from build123d import *

# Parameters (mm, degrees)
SKIZZE1_W                       = 20
SKIZZE1_H                       = 40
AUFSATZ_LINEAR_AUSTRAGEN1_DEPTH = 300
SCHNITT_LINEAR_AUSTRAGEN1_DEPTH = 304.315017762


with BuildPart() as part:
    # Skizze1 → Aufsatz-Linear austragen1 (new body)
    with BuildSketch(Plane(origin=(0, 0, 0), x_dir=(1, 0, 0), z_dir=(0, 1, 0))):
        with Locations((10, 20)):
            Rectangle(SKIZZE1_W, SKIZZE1_H)
    extrude(amount=AUFSATZ_LINEAR_AUSTRAGEN1_DEPTH)

    # Skizze2 → Schnitt-Linear austragen1 (cut, through all)
    with BuildSketch(Plane(origin=(0, 300, 0), x_dir=(1, 0, 0), z_dir=(0, 1, 0))):
        Polygon((3, 30), (0, 33), (0, 27), align=None)
        Polygon((13, 40), (7, 40), (10, 37), align=None)
        Polygon((20, 27), (20, 33), (17, 30), align=None)
        Polygon((13, 20), (10, 17), (7, 20), align=None)
        Polygon((7, 20), (10, 23), (13, 20), align=None)
        Polygon((20, 7), (20, 13), (17, 10), align=None)
        Polygon((3, 10), (0, 13), (0, 7), align=None)
        Polygon((10, 3), (7, 0), (13, 0), align=None)
    extrude(amount=-SCHNITT_LINEAR_AUSTRAGEN1_DEPTH, mode=Mode.SUBTRACT)


solid = part.part
Could you check a few things on this model? Use its own coordinates, in mm. Coordinates: 2 decimals unless noted, no trailing zeros. Loops run counter-clockwise (first coordinate to the right, second up) from the corner with the lowest first, then second, coordinate; pieces in that order, holes last.
1. I need wall thicknesses on L1, parallel to X at y = 138, z = -20; L2, parallel to Z at x = 1.75, y = 84.5; L3, parallel to Z at x = 8, y = 120.5. Which ranges of each line are inside material? Lowest first, please.
2. For P1, Ø1, axis at x = 9.5, y = 89, coming from the +Z side; P2, Ø1, axis at x = 8.5, y = 57, coming from the +Z side, each with a flat end and sliding along its axis, tell me the tip position at first contact or that it passes through.
3. Imagine slicing it at A-A (y = 276.5). Please give me the cut outline in (x, z), and give its area (3 significant figures).
Computed values:
1. L1: x = 0 to 7, 13 to 20
1. L2: z = -40 to -31.25, -28.75 to -11.25, -8.75 to 0
1. L3: z = -39 to -21, -19 to -1
2. P1: stops at z = -2
2. P2: stops at z = -1
3. outline: (0, -40) - (7, -40) - (10, -37) - (13, -40) - (20, -40) - (20, -33) - (17, -30) - (20, -27) - (20, -13) - (17, -10) - (20, -7) - (20, 0) - (13, 0) - (10, -3) - (7, 0) - (0, 0) - (0, -7) - (3, -10) - (0, -13) - (0, -27) - (3, -30) - (0, -33) - close; hole (7, -20) - (10, -23) - (13, -20) - (10, -17) - close
3. area: 728 mm2
